Autodesk Inventor part; units mm, degrees
ref_plane "YZ Plane" through (0, 0, 0) normal (1, 0, 0) x (0, 1, 0)
ref_plane "XZ Plane" through (0, 0, 0) normal (0, 1, 0) x (-1, 0, 0)
ref_plane "XY Plane" through (0, 0, 0) normal (0, 0, 1) x (1, 0, 0)
sketch "Sketch1" plane through (0, 0, 0) normal (1, 0, 0) x (0, 1, 0)
  line L0 (0, 0) -> (56.134, 0)
  line L1 (56.134, 0) -> (56.134, -3.175)
  line L2 (56.134, -3.175) -> (0, -3.175)
  line L3 (0, -3.175) -> (0, 0)
  dimension "d0" = 56.134
  dimension "d1" = 3.175
extrude "Extrusion1" add sketch "Sketch1" along normal blind 25.4
sketch "Sketch2" plane through (0, 56.134, 0) normal (0, 1, 0) x (1, 0, 0)
  line L0 (0, 3.175) -> (25.4, 3.175)
  line L1 (11.1125, 3.175) -> (11.1125, 0)
  line L2 (14.2875, 0) -> (14.2875, 3.175)
  line L3 (11.1125, 3.175) -> (14.2875, 3.175)
  line L4 (14.2875, 0) -> (11.1125, 0)
  line L5 (0, 3.175) -> (25.4, 3.175)
  line L6 (0, 0) -> (0, 3.175)
  line L7 (0, 0) -> (25.4, 0)
  line L8 (25.4, 3.175) -> (25.4, 0)
  line L9 (0, 3.175) -> (25.4, 3.175)
  line L10 (14.2875, 0) -> (11.1125, 0)
sketch "Sketch3" plane through (0, 0, 0) normal (0, 0, 1) x (1, 0, 0)
  line L0 (14.2875, 56.134) -> (11.1125, 57.2894)
  line L1 (11.1125, 57.2894) -> (11.1125, 56.134)
  line L2 (0, 56.134) -> (25.4, 56.134)
  point P0 (0, 0)
extrude "Extrusion2" add sketch "Sketch3" against normal blind 3.175
sketch "Sketch4" plane through (14.2875, 56.134, 0) normal (0.341963, 0.9397134, 0) x (0.9397134, -0.341963, 0)
  line L0 (0, 3.175) -> (0, 0)
  line L1 (-3.3787, 0) -> (-3.3787, 3.175)
  line L2 (0, 3.175) -> (-3.3787, 3.175)
  line L3 (-3.3787, 3.175) -> (-3.3787, 0)
  line L4 (-3.3787, 0) -> (0, 0)
  line L5 (0, 0) -> (0, 3.175)
  point P0 (5.7696, 0)
extrude "Extrusion3" add sketch "Sketch4" along normal blind 25.4
sketch "Sketch5" plane through (22.9734, 80.0027, 0) normal (0.341963, 0.9397134, 0) x (0.9397134, -0.341963, 0)
  point P0 (5.7696, 0)
sketch "Sketch6" plane through (0, 0, -3.175) normal (0, 0, -1) x (-1, 0, 0)
  line L0 (-19.7984, 81.1581) -> (-22.9734, 80.0027)
  line L1 (-19.7984, 81.1581) -> (-22.9734, 81.1581)
  line L2 (-22.9734, 81.1581) -> (-22.9734, 80.0027)
  point P0 (0, 0)
extrude "Extrusion4" add sketch "Sketch6" against normal blind 3.175
sketch "Sketch7" plane through (0, 0, 0) normal (0, 0, 1) x (1, 0, 0)
  line L0 (0, 56.134) -> (11.1125, 56.134)
  line L1 (11.1125, 56.134) -> (11.1125, 0)
  line L2 (0, 0) -> (25.4, 0)
  line L3 (11.1125, 0) -> (0, 0)
  line L4 (0, 0) -> (0, 56.134)
  line L5 (0, 0) -> (0, 56.134)
  line L6 (14.2875, 56.134) -> (25.4, 56.134)
  line L7 (14.2875, 56.134) -> (14.2875, 0)
  line L8 (25.4, 56.134) -> (25.4, 0)
  line L9 (25.4, 0) -> (25.4, 56.134)
extrude "Extrusion5" cut sketch "Sketch7" against normal blind 25.4
sketch "Sketch8" plane through (11.1125, 0, 0) normal (0, 0, 1) x (1, 0, 0)
  line L0 (3.175, 56.134) -> (11.8609, 80.0027)
  line L1 (3.175, 56.134) -> (0, 56.134)
  line L2 (0, 0) -> (0, 57.2894)
  line L3 (0, 0) -> (3.175, 0)
  line L4 (3.175, 0) -> (0, 0)
  line L5 (3.175, 56.134) -> (3.175, 0)
  point P0 (-11.1125, 0)
extrude "Extrusion6" add sketch "Sketch8" along normal blind 25.4
sketch "Sketch9" plane through (11.1125, 0, -3.175) normal (0, 0, -1) x (-1, 0, 0)
  line L0 (0, 0) -> (-3.175, 0)
  line L1 (-3.175, 56.134) -> (-3.175, 0)
  line L2 (0, 0) -> (-3.175, 0)
  line L3 (-3.175, 0) -> (-3.175, 56.134)
  line L4 (-3.175, 56.134) -> (0, 56.134)
  line L5 (0, 56.134) -> (0, 0)
  point P0 (11.1125, 0)
extrude "Extrusion7" add sketch "Sketch9" along normal blind 25.4
properties part number "ClawPaddle"
For this review, take the finished solid that the model builds, in its own axes (mm). A direction names the side the tool comes from. Coordinates: 2 decimals unless noted, no trailing zeros. Loops run counter-clockwise (first coordinate to the right, second up) from the corner with the lowest first, then second, coordinate; pieces in that order, holes last. Notation, with made-up numbers: (45, 10.25) -> (100, 10.25) arc R4 cw to (100, 17.25) -> close; hole circle Ø7 at (14, 14). An arc over 180 degrees is marked (long way). Write each question's results on one line, items separated by ' | '.
Q1. To check wall thickness, follow line 1 along X through (y, z) = (41, 0); line 2 along Y through (x, z) = (12.5, -4.5); line 3 along Z through (x, y) = (16.5, 65) (3 decimals). State the ranges of each line that lie inside material, in increasing order. Write a range as [from, to].
Taken from the geometry:
line 1: [11.11, 14.29] | line 2: [0, 56.13] | line 3: [-3.175, 0]
Q2. Add section A-A, the plane y = 12.5. State the section outline as (x, z) points (1 decimal).
Taken from the geometry:
outline: (11.1, -28.6) -> (14.3, -28.6) -> (14.3, 25.4) -> (11.1, 25.4) -> close
Q3. Machinability: for faces 1 (the flat face through (15.395, 69.057, -1.565)), 2 (the flat face through (17, 68, 0)), 3 (the flat face through (17, 68, -3.175)), which of the approach directions +Z, -Z, +X, -X, +Y, -Y give a long, thin tool a straight path to every point of the face, cutting with its end or side? Answer none if there is none.
Taken from the geometry:
face 1: +Z, -Z, -X, +Y | face 2: +Z, +X, -X, +Y | face 3: -Z, +X, -X, +Y
Q4. For pin 1 Ø5 at (y, z) = (11, -23) entering from +X; pin 2 Ø2.5 at (x, z) = (12.5, 11) entering from +Y; pin 3 Ø6 at (x, y) = (20, 68) entering from -Z (3 decimals), all flat-tipped, find the tip position at first contact; note any pin that passes through.
Taken from the geometry:
pin 1: x = 14.29 | pin 2: y = 56.13 | pin 3: z = -3.175
Q5. Add section B-B, the plane x = 12. State the section outline as (y, z) points (3 decimals).
Taken from the geometry:
outline: (0, -28.575) -> (56.134, -28.575) -> (56.134, -3.175) -> (59.728, -3.175) -> (59.728, 0) -> (56.134, 0) -> (56.134, 25.4) -> (0, 25.4) -> close
Q6. Add section C-C, the plane z = -17.5. State the section outline as (x, y) points.
Taken from the geometry:
outline: (11.11, 0) -> (14.29, 0) -> (14.29, 56.13) -> (11.11, 56.13) -> close
